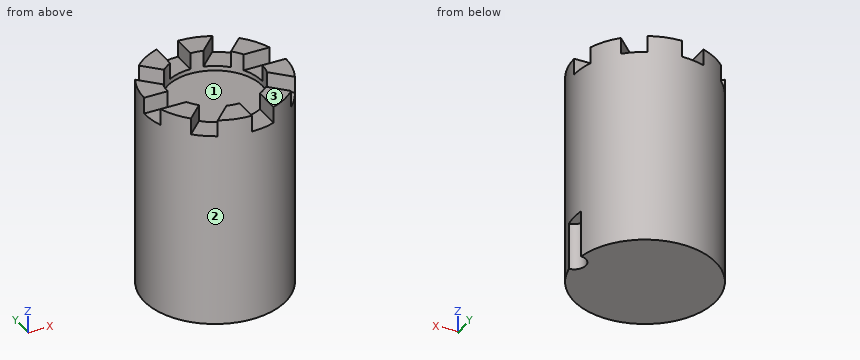
from build123d import *

# Parameters (mm, degrees)
CYLINDER002_R     = 5
CYLINDER002_DEPTH = 20
BOX_W             = 20
BOX_H             = 10
BOX_DEPTH         = 10
ARRAY_COUNT       = 8
CYLINDER001_R     = 20
CYLINDER001_DEPTH = 10
CYLINDER_R        = 30
CYLINDER_DEPTH    = 90


with BuildPart() as cilindro:
    # Cylinder002 → Cylinder002 (new body)
    with BuildSketch(Plane(origin=(30, 0, 0), x_dir=(1, 0, 0), z_dir=(0, 0, 1))):
        Circle(CYLINDER002_R)
    extrude(amount=CYLINDER002_DEPTH)


with BuildPart() as array:
    # Box → Box (new body)
    with BuildSketch(Plane(origin=(13, 0, 83), x_dir=(1, 0, 0), z_dir=(0, 0, 1))):
        with Locations((10, 5)):
            Rectangle(BOX_W, BOX_H)
    extrude(amount=BOX_DEPTH)

    # Array: Array ×8 about axis
    array_axis = Axis((0, 0, 0), (0, 0, 1))


with BuildPart() as array_1:
    add(array.part)
    for i in range(1, ARRAY_COUNT):
        add(array.part.rotate(array_axis, i * 360 / ARRAY_COUNT))


with BuildPart() as cylinder001:
    # Cylinder001 → Cylinder001 (new body)
    with BuildSketch(Plane.XY.offset(81)):
        Circle(CYLINDER001_R)
    extrude(amount=CYLINDER001_DEPTH)


with BuildPart() as cut002:
    # Cylinder → Cylinder (new body)
    with BuildSketch(Plane.XY):
        Circle(CYLINDER_R)
    extrude(amount=CYLINDER_DEPTH)

    # Cut: cut Cylinder001
    add(cylinder001.part, mode=Mode.SUBTRACT)

    # Cut001: cut Array
    add(array_1.part, mode=Mode.SUBTRACT)

    # Cut002: cut Cilindro
    add(cilindro.part, mode=Mode.SUBTRACT)


solid = cut002.part
Source: CAD feature listing. Evaluate the final solid. Frame: model axes, mm. Face numbers are marked on the shaded views. Round coordinates to 2 decimals unless told otherwise and drop trailing zeros. Loops run counter-clockwise (first coordinate to the right, second up) from the corner with the lowest first, then second, coordinate; pieces in that order, holes last. Notation, with made-up numbers: (9.5, 61.25) - (59.5, 61.25) arc R25 ccw to (59.5, 77.25) - close; hole circle Ø1 at (-21, -17). An arc over 180 degrees is marked (long way). Write item = value, one per line. Start each with the question number.
Item 1: Section query A-A on y = 25.5. Output: boundary loops of the cut face in (x, z), plus the area to 3 significant figures.
Item 2: Section query C-C on x = 7. Output: boundary loops of the cut face in (y, z) (3 decimals), plus the area to 3 significant figures.
Item 3: Material intervals for line 1 (Z direction, x = -5, y = -4.5); line 2 (Y direction, x = 12, z = 84); line 3 (Z direction, x = -13.5, y = -15), sorted ascending.
Item 4: Section query D-D on z = 17. Output: boundary loops of the cut face in (x, y).
Item 5: First-contact query: pin 1 Ø5 at (x, y) = (-6.5, 23) entering from +Z; pin 2 Ø1 at (y, z) = (15.5, 52) entering from +X; pin 3 Ø2 at (y, z) = (-22.5, 88) entering from -X. Flat tips, straight axial feed; report the tip coordinate or a pass-through.
Item 6: Mould query, pull axis Y, two halves, no side actions, for the marked faces 1, 2 and 3. Classes: released by +Y, released by -Y, zero draft, split by the parting line, or undercut.
Item 7: Section query B-B on z = 54. Output: boundary loops of the cut face in (x, y).
Results list:
q1.outline = (-15.8, 0) - (15.8, 0) - (15.8, 83) - (11.36, 83) - (11.36, 90) - (0, 90) - (0, 83) - (-10, 83) - (-10, 90) - (-15.8, 90) - close
q1.area = 2,740 mm²
q2.outline = (-29.172, 0) - (29.172, 0) - (29.172, 90) - (21.142, 90) - (21.142, 83) - (18.735, 83) - (18.735, 81) - (-18.735, 81) - (-18.735, 83) - (-29.172, 83) - close
q2.area = 4,820 mm²
q3.line_1 = 0 to 81
q3.line_2 = -27.5 to -16, 26.14 to 27.5
q3.line_3 = 0 to 83
q4.outline = (29.58, -4.98) arc R5 cw to (29.58, 4.98) arc R30 ccw (long way) to start
q5.pin_1 = 83
q5.pin_2 = 25.98
q5.pin_3 = -9.36
q6.face_1 = undercut
q6.face_2 = split by the parting line
q6.face_3 = zero draft
q7.outline = circle Ø60 at (0, 0)
